Autodesk Inventor part; units mm, degrees
ref_plane "YZ Plane" through (0, 0, 0) normal (1, 0, 0) x (0, 1, 0)
ref_plane "XZ Plane" through (0, 0, 0) normal (0, 1, 0) x (-1, 0, 0)
ref_plane "XY Plane" through (0, 0, 0) normal (0, 0, 1) x (1, 0, 0)
sketch "Sketch1" plane through (0, 0, 0) normal (0, 1, 0) x (-1, 0, 0)
  circle A0 centre (0, 0) radius 2
  dimension "d0" = 4
extrude "Extrusion1" add sketch "Sketch1" along normal blind 16
sketch "Sketch2" plane through (0, 16, 0) normal (0, 1, 0) x (1, 0, 0)
  circle A0 centre (0, 0) radius 2
  circle A1 centre (0, 0) radius 3.5
  dimension "d3" = 7
extrude "Extrusion2" add sketch "Sketch2" along normal blind 4 contours A0 | A1
sketch "Sketch3" plane through (0, 20, 0) normal (0, 1, 0) x (1, 0, 0)
  circle A0 centre (0, 0) radius 3.5
  line L0 (0, 1.8475) -> (1.6, 0.9238)
  line L1 (1.6, 0.9238) -> (1.6, -0.9238)
  line L2 (1.6, -0.9238) -> (0, -1.8475)
  line L3 (0, -1.8475) -> (-1.6, -0.9238)
  line L4 (-1.6, -0.9238) -> (-1.6, 0.9238)
  line L5 (-1.6, 0.9238) -> (0, 1.8475)
  dimension "d6" = 1.6
extrude "Extrusion3" cut sketch "Sketch3" against normal blind 3 contours L0 L1 L2 L3 L4 L5
thread "Thread1"
chamfer "Chamfer1" distance 0.25 angle 45 1 edges at (2, 0, 0)
properties part number "M4x14SHCS"
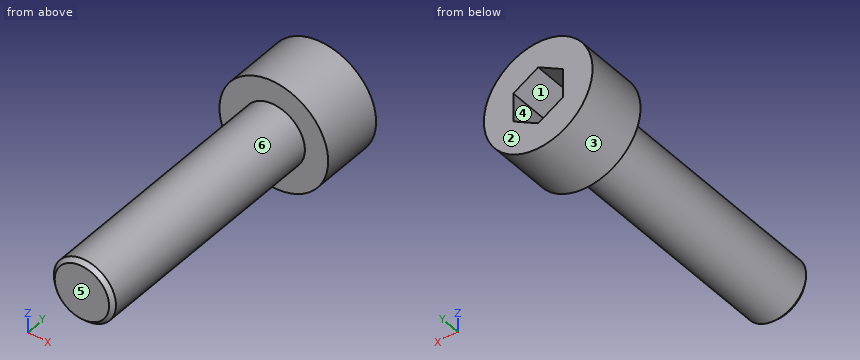
Can you work these out from the model? Positions are in its coordinate system, mm. Face numbers are marked on the shaded views. A direction names the side the tool comes from. Give positions to 0.01 mm unless a question says otherwise; leave off trailing zeros. Write each loop counter-clockwise with the first axis right and the second up, starting at its lowest first coordinate (ties: lowest second). Pieces come first, ordered by that corner, then holes. Notation, with made-up numbers: (69.25, -9) -> (99.25, -9) arc R17 cw to (99.25, 24) -> close; hole circle Ø7 at (-13, 73). An arc over 180 degrees is marked (long way). Answer as a JSON object with one key per item and string values. Group by question number.
Item 1: Suppose I cut it at B-B (y = 6). Please give me the cut outline in (x, z).
Item 2: Suppose I cut it at C-C (z = -2.75). Please give me the cut outline in (x, y), plus the area to 3 significant figures.
Item 3: Suppose I cut it at D-D (z = 3.25). Please give me the cut outline in (x, y).
Item 4: We'd pull the mould along X, two halves only. Please class the marked faces 1, 2 and 3: +X half, -X half, draft (parallel to the pull), parting line (faces both ways), or undercut.
Item 5: Please list where these lines run through material, in increasing order: line 1 (Y direction, x = 1.5, z = -1.75); line 2 (Z direction, x = -0.75, y = 2.25); line 3 (Z direction, x = -1.5, y = 19.25). Write a range as [from, to].
Item 6: For the marked faces 4, 5 and 6, which set-ups out of +Z, -Z, +X, -X, +Y, -Y let a thin tool reach every point of the face, with its end or its side?
Item 7: I'm going to push flat-ended pins straight in: P1, Ø4, axis at x = -0.5, y = 2.5, coming from the -Z side; P2, Ø1.5, axis at x = -2.5, z = 1.5, coming from the -Y side; P3, Ø0.6, axis at y = 18, z = 0.5, coming from the -X side. Where does each tip first touch, or does it pass through?
Item 8: Suppose I cut it at A-A (z = 0). Please give me the cut outline in (x, y).
Findings:
{
 "1": {"outline": "circle Ø4 at (0, 0)"},
 "2": {"outline": "(-2.17, 16) -> (2.17, 16) -> (2.17, 20) -> (-2.17, 20) -> close", "area": "17.3 mm²"},
 "3": {"outline": "(-1.3, 16) -> (1.3, 16) -> (1.3, 20) -> (-1.3, 20) -> close"},
 "4": {"face 1": "undercut", "face 2": "draft", "face 3": "parting line"},
 "5": {"line 1": "y = [16, 20]", "line 2": "z = [-1.85, 1.85]", "line 3": "z = [-3.16, -0.98], [0.98, 3.16]"},
 "6": {"face 4": "+Y", "face 5": "+Z, -Z, +X, -X, -Y", "face 6": "-Y"},
 "7": {"P1": "stops at z = -2", "P2": "stops at y = 16", "P3": "stops at x = -3.49"},
 "8": {"outline": "(-3.5, 16) -> (-2, 16) -> (-2, 0.25) -> (-1.75, 0) -> (1.75, 0) -> (2, 0.25) -> (2, 16) -> (3.5, 16) -> (3.5, 20) -> (1.6, 20) -> (1.6, 17) -> (-1.6, 17) -> (-1.6, 20) -> (-3.5, 20) -> close"}
}
